```python
from build123d import *

# Parameters (mm, degrees)
F0_R     = 11.05
F1_DEPTH = 6.35
F2_SIZE  = 0.4


with BuildPart() as f1:
    # F0 (on Top) → F1 (new body)
    with BuildSketch(Plane.XY):
        with BuildLine():
            Line((-9.577975, 23.157779), (-13.804711, 26.316489))
            ThreePointArc((-13.804711, 26.316489), (-37.239092, 21.5), (-29.693104, -1.203014))
            Line((-29.693104, -1.203014), (-24.844213, -3.28412))
            ThreePointArc((-24.844213, -3.28412), (-17.298224, -9.987134), (-15.266238, -19.873659))
            Line((-15.266238, -19.873659), (-15.888393, -25.113475))
            ThreePointArc((-15.888393, -25.113475), (0, -43), (15.888393, -25.113475))
            Line((15.888393, -25.113475), (15.266238, -19.873659))
            ThreePointArc((15.266238, -19.873659), (17.298224, -9.987134), (24.844213, -3.28412))
            Line((24.844213, -3.28412), (29.693104, -1.203014))
            ThreePointArc((29.693104, -1.203014), (37.239092, 21.5), (13.804711, 26.316489))
            Line((13.804711, 26.316489), (9.577975, 23.157779))
            ThreePointArc((9.577975, 23.157779), (0, 19.974269), (-9.577975, 23.157779))
        make_face()
        with Locations((0, -27)):
            Circle(F0_R, mode=Mode.SUBTRACT)
        with Locations((-23.382686, 13.5)):
            Circle(F0_R, mode=Mode.SUBTRACT)
        Circle(F0_R, mode=Mode.SUBTRACT)
        with Locations((23.382686, 13.5)):
            Circle(F0_R, mode=Mode.SUBTRACT)
    extrude(amount=F1_DEPTH)

    # F2
    f2_edges = [f1.edges().sort_by_distance(p)[0] for p in [
        (-11.05, 0, 6.35),
        (-11.05, 0, 0),
        (-11.05, -27, 6.35),
        (-11.05, -27, 0),
        (-34.432686, 13.5, 6.35),
        (-34.432686, 13.5, 0),
        (12.332686, 13.5, 6.35),
        (12.332686, 13.5, 0),
    ]]
    chamfer(f2_edges, length=F2_SIZE)


solid = f1.part
```
Geometry: final body of the model. Coordinates: model frame, mm. A direction names the side the tool comes from. Round coordinates to 2 decimals unless told otherwise and drop trailing zeros. Write each loop counter-clockwise with the first axis right and the second up, starting at its lowest first coordinate (ties: lowest second). Pieces come first, ordered by that corner, then holes.
Item 1: Section query A-A (y = -27). Return loops of the section in (x, z), plus the area to 3 significant figures.
Item 2: Section query B-B (z = 3.75). Return loops of the section in (x, y), plus the area to 3 significant figures.
Item 3: Pin query (flat end, axial travel): P1, Ø2, axis at x = -19.5, z = 5, coming from the -Y side; P2, Ø3, axis at y = -35.5, z = 4.5, coming from the +X side; P3, Ø1.5, axis at y = -16.5, z = 1, coming from the -X side. Return the tip coordinate at first contact, or that it passes through.
Item 4: Section query C-C (y = 13.5). Return loops of the section in (x, z).
Item 5: Section query D-D (y = 0). Return loops of the section in (x, z), plus the area to 3 significant figures.
Item 6: Mould query, pull axis Y, two halves, no side actions, for faces 1 (the face through (9, -9, 6.35)), 2 (the face through (37.424, 21.17, 3.131)), 3 (the face through (17.23, -10.11, 3.13)). Classes: +Y half, -Y half, draft (parallel to the pull), parting line (faces both ways), or undercut.
Item 7: Set-up query: faces 4 (the face through (-11.662, 24.715, 3.131)), 5 (the face through (9, -9, 0)), 6 (the face through (15.58, -22.53, 3.13)). Return all of +Z, -Z, +X, -X, +Y, -Y with unobstructed straight access to the full face (end or side cutting, diameter ignored); none if empty.
Item 8: Material intervals for L1, parallel to X at y = 14, z = 3.75; L2, parallel to Y at x = 0, z = 3.3; L3, parallel to X at y = 6, z = 5.75, sorted ascending.
Completed:
1. outline: (-16, 0) - (-11.45, 0) - (-11.05, 0.4) - (-11.05, 5.95) - (-11.45, 6.35) - (-16, 6.35) - close; (11.05, 0.4) - (11.45, 0) - (16, 0) - (16, 6.35) - (11.45, 6.35) - (11.05, 5.95) - close
1. area: 62.5 mm2
2. outline: (-29.69, -1.2) - (-24.84, -3.28) arc R16 cw to (-15.27, -19.87) - (-15.89, -25.11) arc R16 ccw (long way) to (15.89, -25.11) - (15.27, -19.87) arc R16 cw to (24.84, -3.28) - (29.69, -1.2) arc R16 ccw (long way) to (13.8, 26.32) - (9.58, 23.16) arc R16 cw to (-9.58, 23.16) - (-13.8, 26.32) arc R16 ccw (long way) to start; hole circle Ø22.1 at (-23.38, 13.5); hole circle Ø22.1 at (0, -27); hole circle Ø22.1 at (0, 0); hole circle Ø22.1 at (23.38, 13.5)
2. area: 1,790 mm2
3. P1: stops at y = -8.2
3. P2: stops at x = 14.39
3. P3: stops at x = -15.31
4. outline: (-39.38, 0) - (-34.83, 0) - (-34.43, 0.4) - (-34.43, 5.95) - (-34.83, 6.35) - (-39.38, 6.35) - close; (-12.33, 0.4) - (-11.93, 0) - (11.93, 0) - (12.33, 0.4) - (12.33, 5.95) - (11.93, 6.35) - (-11.93, 6.35) - (-12.33, 5.95) - close; (34.43, 0.4) - (34.83, 0) - (39.38, 0) - (39.38, 6.35) - (34.83, 6.35) - (34.43, 5.95) - close
5. outline: (-31.97, 0) - (-11.45, 0) - (-11.05, 0.4) - (-11.05, 5.95) - (-11.45, 6.35) - (-31.97, 6.35) - close; (11.05, 0.4) - (11.45, 0) - (31.97, 0) - (31.97, 6.35) - (11.45, 6.35) - (11.05, 5.95) - close
5. area: 265 mm2
6. face 1: draft
6. face 2: parting line
6. face 3: undercut
7. face 4: +Z, -Z, +Y
7. face 5: -Z, +X, -X, +Y, -Y
7. face 6: +Z, -Z, +X
8. L1: x = -39.37 to -34.42, -12.34 to 12.34, 34.42 to 39.37
8. L2: y = -43 to -38.05, -15.95 to -11.05, 11.05 to 19.97
8. L3: x = -37.52 to -31.5, -15.27 to -9.28, 9.28 to 15.27, 31.5 to 37.52
